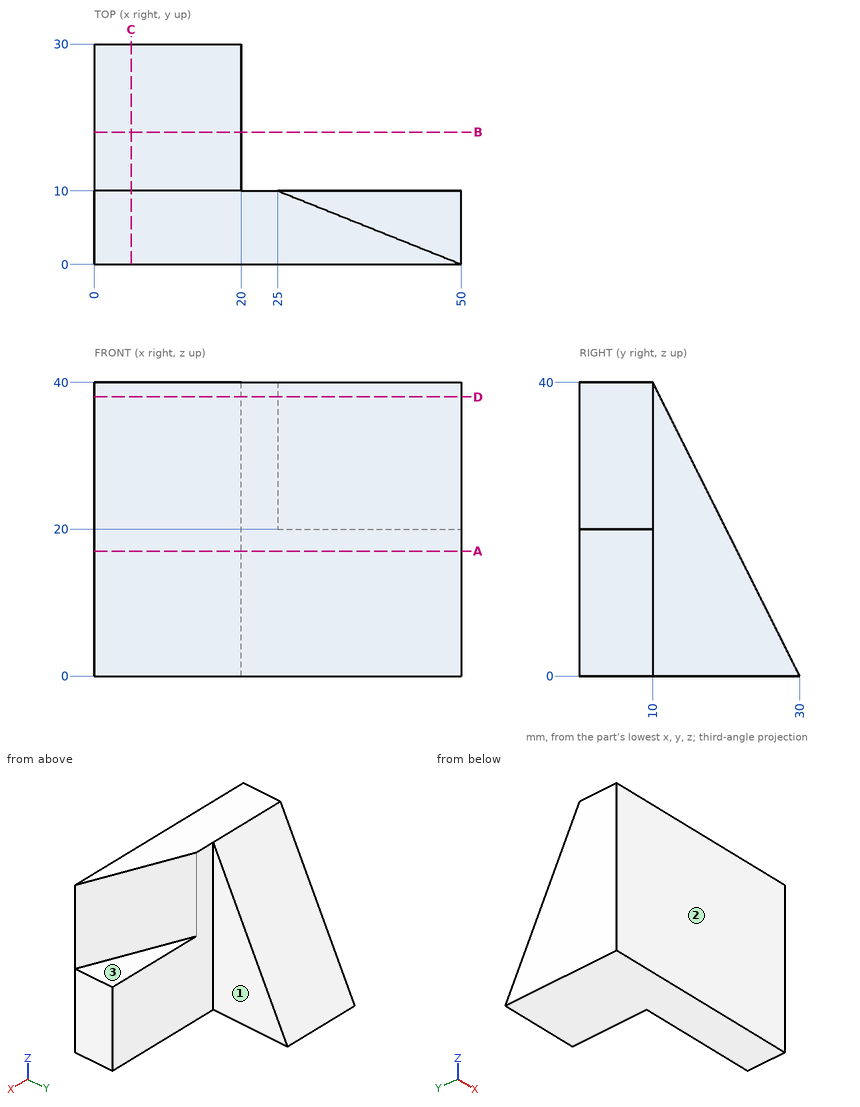
Part print with two shaded views. Sizes in mm from the minimum x, y, z corner. A direction names the side the tool comes from. Give positions to 0.01 mm unless a question says otherwise; leave off trailing zeros. Loops run counter-clockwise (first coordinate to the right, second up) from the corner with the lowest first, then second, coordinate; pieces in that order, holes last. Notation, with made-up numbers: (0, -1.5) -> (9, -1.5) arc R31 ccw to (9, 36.5) -> close; hole circle Ø5 at (88.5, -34). An arc over 180 degrees is marked (long way). One line per question, with ' | ' between items.
Q1. Cut at D-D, the plane z = 38. Write the cut outline in (x, y), plus the area to 3 significant figures.
Filled sheet:
outline: (0, 0) -> (50, 0) -> (25, 10) -> (20, 10) -> (20, 11) -> (0, 11) -> close | area: 395 mm²
Q2. Tool access for the marked faces 1, 2 and 3: list every direction of +Z, -Z, +X, -X, +Y, -Y with a clear straight run to the whole face (end or side of a thin tool).
Filled sheet:
face 1: +Z, -Z, +X, +Y | face 2: +Z, -Z, +X, -X, -Y | face 3: +Z, +X, +Y
Q3. Drop flat-ended pins along their axis: pin 1 (2 mm diameter, centred on x = 29.5, z = 24, fed in from +Y); pin 2 (12 mm diameter, centred on x = 11, z = 5, fed in from +Y); pin 3 (1.5 mm diameter, centred on y = 19.5, z = 16, fed in from +X). Give the stop position or say it passes through.
Filled sheet:
pin 1: stops at y = 8.6 | pin 2: stops at y = 30 | pin 3: stops at x = 20
Q4. Cut at A-A, the plane z = 17. Write the cut outline in (x, y).
Filled sheet:
outline: (0, 0) -> (50, 0) -> (50, 10) -> (20, 10) -> (20, 21.5) -> (0, 21.5) -> close
Q5. Drill centre lines: line 1 along Y through (x, z) = (48.5, 14); line 2 along X through (y, z) = (11.25, 24.5); line 3 along Y through (x, z) = (35, 21.5). Where is each one in solid material? Low to high. Write a range as [from, to].
Filled sheet:
line 1: y = [0, 10] | line 2: x = [0, 20] | line 3: y = [0, 6]
Q6. Cut at B-B, the plane y = 18. Write the cut outline in (x, z), plus the area to 3 significant figures.
Filled sheet:
outline: (0, 0) -> (20, 0) -> (20, 24) -> (0, 24) -> close | area: 480 mm²
Q7. Cut at C-C, the plane x = 5. Write the cut outline in (y, z).
Filled sheet:
outline: (0, 0) -> (30, 0) -> (10, 40) -> (0, 40) -> close
